from build123d import *

# Parameters (mm, degrees)
SKETCH1_W               = 107.95
SKETCH1_H               = 63.5
BOSS_EXTRUDE5_DEPTH     = 133.35
SKETCH5_OUTSIDE_W       = 146.538
SKETCH5_OUTSIDE_H       = 102.088
SKETCH5_OUTSIDE_W_2     = 107.95
SKETCH5_OUTSIDE_H_2     = 63.5
CUT_EXTRUDE4_DEPTH      = 128.27
SKETCH6_W               = 107.95
SKETCH6_H               = 63.5
SKETCH6_R               = 12.7
BOSS_EXTRUDE6_DEPTH     = 2.54
CUT_EXTRUDE6_REACH      = 186.801
CUT_EXTRUDE6_END_RADIUS = 25.4
SKETCH8_R               = 10.16


with BuildPart() as part:
    # Sketch1 → Boss-Extrude5 (new body)
    with BuildSketch(Plane.XY):
        with Locations((53.975, 31.75)):
            Rectangle(SKETCH1_W, SKETCH1_H)
    extrude(amount=BOSS_EXTRUDE5_DEPTH)

    # Sketch5 outside → Cut-Extrude4 (cut)
    # profile 1 of 2: a face of its own
    with BuildSketch(Plane.XY.offset(133.35)):
        with Locations((53.975, 31.75)):
            Rectangle(SKETCH5_OUTSIDE_W, SKETCH5_OUTSIDE_H)
        with Locations((53.975, 31.75)):
            Rectangle(SKETCH5_OUTSIDE_W_2, SKETCH5_OUTSIDE_H_2, mode=Mode.SUBTRACT)
    # profile 2 of 2: a face of its own
    with BuildSketch(Plane.XY.offset(133.35)):
        with BuildLine():
            Line((31.75, 60.325), (76.2, 60.325))
            ThreePointArc((76.2, 60.325), (101.6, 34.925), (76.2, 9.525))
            Line((76.2, 9.525), (31.75, 9.525))
            ThreePointArc((31.75, 9.525), (6.35, 34.925), (31.75, 60.325))
        make_face()
    extrude(amount=-CUT_EXTRUDE4_DEPTH, mode=Mode.SUBTRACT)

    # Sketch6 → Boss-Extrude6 (add)
    with BuildSketch(Plane.XY.offset(133.35)):
        with Locations((53.975, 31.75)):
            Rectangle(SKETCH6_W, SKETCH6_H)
        with Locations((53.975, 34.925)):
            Circle(SKETCH6_R, mode=Mode.SUBTRACT)
    extrude(amount=BOSS_EXTRUDE6_DEPTH)

    # Cut-Extrude6: up to this cylinder (the profile starts outside it)
    cut_extrude6_end = Plane(origin=(76.2, 34.925, 64.77), z_dir=(0, 0, 1)) * Cylinder(CUT_EXTRUDE6_END_RADIUS, 516.842, mode=Mode.PRIVATE)
    # Sketch8 → Cut-Extrude6 (cut, up to the surface)
    with BuildSketch(Plane.XZ.offset(-63.5), mode=Mode.PRIVATE) as cut_extrude6_sk1:
        with Locations(Location((88.9, 19.05, 0), (0, 0, 90))):
            Circle(SKETCH8_R)
    cut_extrude6_tool1 = extrude(cut_extrude6_sk1.sketch, amount=CUT_EXTRUDE6_REACH, mode=Mode.PRIVATE) - cut_extrude6_end
    add(cut_extrude6_tool1.solids().sort_by_distance((88.9, 63.5, 19.05))[0], mode=Mode.SUBTRACT)
    # Sketch8 → Cut-Extrude6 (cut, up to the surface)
    with BuildSketch(Plane.XZ.offset(-63.5), mode=Mode.PRIVATE) as cut_extrude6_sk2:
        with Locations(Location((88.9, 110.49, 0), (0, 0, 90))):
            Circle(SKETCH8_R)
    cut_extrude6_tool2 = extrude(cut_extrude6_sk2.sketch, amount=CUT_EXTRUDE6_REACH, mode=Mode.PRIVATE) - cut_extrude6_end
    add(cut_extrude6_tool2.solids().sort_by_distance((88.9, 63.5, 110.49))[0], mode=Mode.SUBTRACT)


solid = part.part
Input: part model. Units: mm. Frame: model coordinates. A direction names the side the tool comes from. Give positions to 0.01 mm unless a question says otherwise; leave off trailing zeros. Write each loop counter-clockwise with the first axis right and the second up, starting at its lowest first coordinate (ties: lowest second). Pieces come first, ordered by that corner, then holes. Notation, with made-up numbers: (29.5, -21.5) -> (80.5, -21.5) arc R22 cw to (80.5, -1.5) -> close; hole circle Ø7 at (22, 79). An arc over 180 degrees is marked (long way). Use one line per item in the form item = value. Start each with the question number.
1) Section query C-C on y = 53.5. Return the cut outline in (x, z), then the cut area to 3 significant figures.
2) Set-up query: faces 1 (the cylindrical face through (66.1, 38.7, 134.6)), 2 (the cylindrical face through (98.82, 58.76, 108.29)), 3 (the cylindrical face through (101.594, 35.484, 70.113)). Return all of +Z, -Z, +X, -X, +Y, -Y with unobstructed straight access to the full face (end or side cutting, diameter ignored); none if empty.
3) Section query D-D on x = 28.5. Return the cut outline in (y, z), then the cut area to 3 significant figures.
4) Draft query along Z for faces 4 (the flat face through (53, 63.5, 67)), 5 (the flat face through (54, 60.325, 70)), 6 (the cylindrical face through (98.82, 58.76, 16.85)), 7 (the flat face through (41, 32, 135.89)). Return one class per face: pulls with the +Z half, pulls with the -Z half, needs draft (parallel to the pull), parting line crosses it, or undercut.
5) Ray query, probe 1 along Z at (x, y) = (93.5, 38); probe 2 along Y at (x, z) = (69, 74) (3 decimals); probe 3 along X at (y, z) = (27, 31.5). Return the intervals inside material, ascending. Write a range as from..to.
6) Section query B-B on x = 88.9. Return the cut outline in (y, z).
7) Pin query (flat end, axial travel): pin 1 (12 mm diameter, centred on x = 88.9, z = 19.05, fed in from +Y); pin 2 (15 mm diameter, centred on x = 72, y = 35, fed in from -Z). Return the tip coordinate at first contact, or that it passes through.
8) Section query A-A on z = 125. Return the cut outline in (x, y) (3 decimals).
Outcome:
q1.outline = (0, 0) -> (107.95, 0) -> (107.95, 135.89) -> (0, 135.89) -> close; hole (14.43, 5.08) -> (93.52, 5.08) -> (93.52, 10) arc R10.16 ccw to (93.52, 28.1) -> (93.52, 101.44) arc R10.16 ccw to (93.52, 119.54) -> (93.52, 133.35) -> (14.43, 133.35) -> close
q1.area = 4,380 mm^2
q2.face_1 = +Z
q2.face_2 = +Y
q2.face_3 = none
q3.outline = (0, 0) -> (63.5, 0) -> (63.5, 135.89) -> (0, 135.89) -> close; hole (9.73, 5.08) -> (60.12, 5.08) -> (60.12, 133.35) -> (9.73, 133.35) -> close
q3.area = 2,170 mm^2
q4.face_4 = needs draft
q4.face_5 = undercut
q4.face_6 = undercut
q4.face_7 = pulls with the +Z half
q5.probe_1 = 0..5.08, 133.35..135.89
q5.probe_2 = 0..9.525, 60.325..63.5
q5.probe_3 = 0..7.62, 100.33..107.95
q6.outline = (0, 0) -> (63.5, 0) -> (63.5, 8.89) -> (56.92, 8.89) -> (56.92, 5.08) -> (12.93, 5.08) -> (12.93, 133.35) -> (56.92, 133.35) -> (56.92, 120.65) -> (63.5, 120.65) -> (63.5, 135.89) -> (0, 135.89) -> close; (56.92, 29.21) -> (63.5, 29.21) -> (63.5, 100.33) -> (56.92, 100.33) -> close
q7.pin_1 = 17.74
q7.pin_2 = 0
q8.outline = (0, 0) -> (107.95, 0) -> (107.95, 63.5) -> (0, 63.5) -> close; hole (31.75, 9.525) -> (76.2, 9.525) arc R25.4 ccw to (76.2, 60.325) -> (31.75, 60.325) arc R25.4 ccw to start
